from build123d import *

# Parameters (mm, degrees)
F1_DEPTH = 63.5
F4_DEPTH = 16
F5_DEPTH = 13


with BuildPart() as f1:
    # F0 (on Top) → F1 (new body)
    with BuildSketch(Plane.XY):
        with BuildLine():
            Line((-9.75, 5.612486), (-9.75, -5.612486))
            ThreePointArc((-9.75, -5.612486), (0, -11.25), (9.75, -5.612486))
            Line((9.75, -5.612486), (9.75, 5.612486))
            ThreePointArc((9.75, 5.612486), (0, 11.25), (-9.75, 5.612486))
        make_face()
        with BuildLine():
            ThreePointArc((8.75, -5.338539), (0, -10.25), (-8.75, -5.338539))
            Line((-8.75, -5.338539), (-8.75, 5.338539))
            ThreePointArc((-8.75, 5.338539), (0, 10.25), (8.75, 5.338539))
            Line((8.75, 5.338539), (8.75, -5.338539))
        make_face(mode=Mode.SUBTRACT)
    extrude(amount=F1_DEPTH)

    # F3 (on mid) → F4 (join, symmetric)
    with BuildSketch(Plane.XY.offset(31.75)):
        with BuildLine():
            Line((10.45, -5.796551), (10.45, 5.796551))
            ThreePointArc((10.45, 5.796551), (0, 11.95), (-10.45, 5.796551))
            Line((-10.45, 5.796551), (-10.45, -5.796551))
            ThreePointArc((-10.45, -5.796551), (0, -11.95), (10.45, -5.796551))
        make_face()
        with BuildLine():
            ThreePointArc((-9.75, 5.612486), (0, 11.25), (9.75, 5.612486))
            Line((9.75, 5.612486), (9.75, -5.612486))
            ThreePointArc((9.75, -5.612486), (0, -11.25), (-9.75, -5.612486))
            Line((-9.75, -5.612486), (-9.75, 5.612486))
        make_face(mode=Mode.SUBTRACT)
    extrude(amount=F4_DEPTH, both=True)

    # F3 (on mid) → F5 (cut, symmetric)
    with BuildSketch(Plane.XY.offset(31.75)):
        with BuildLine():
            Line((10.45, -5.796551), (10.45, 5.796551))
            ThreePointArc((10.45, 5.796551), (0, 11.95), (-10.45, 5.796551))
            Line((-10.45, 5.796551), (-10.45, -5.796551))
            ThreePointArc((-10.45, -5.796551), (0, -11.95), (10.45, -5.796551))
        make_face()
        with BuildLine():
            ThreePointArc((-9.75, 5.612486), (0, 11.25), (9.75, 5.612486))
            Line((9.75, 5.612486), (9.75, -5.612486))
            ThreePointArc((9.75, -5.612486), (0, -11.25), (-9.75, -5.612486))
            Line((-9.75, -5.612486), (-9.75, 5.612486))
        make_face(mode=Mode.SUBTRACT)
    extrude(amount=F5_DEPTH, both=True, mode=Mode.SUBTRACT)


solid = f1.part
Could you check a few things on this model? Use its own coordinates, in mm. A direction names the side the tool comes from. Give positions to 0.01 mm unless a question says otherwise; leave off trailing zeros. Loops run counter-clockwise (first coordinate to the right, second up) from the corner with the lowest first, then second, coordinate; pieces in that order, holes last. Notation, with made-up numbers: (30, 75.5) -> (86, 75.5) arc R13 cw to (86, 84.5) -> close; hole circle Ø5 at (21, -15). An arc over 180 degrees is marked (long way). Return JSON: item names as keys, results as strings.
Item 1: Which directions (+Z, -Z, +X, -X, +Y, -Y) give clear straight access to the entire face, cutting with the end or side of a thin tool? Please do faces 5 (the flat face through (-9.75, 0, 56)), 6 (the flat face through (-10, -1, 18.75)), 7 (the cylindrical face through (0.15, -10.25, 31.31)), 8 (the flat face through (-10, -1, 47.75)).
Geometry results:
{"face 5": "+Z, -X, +Y, -Y", "face 6": "none", "face 7": "+Z, -Z", "face 8": "+Z"}
Item 2: If we section it at B-B on z = 53: List the corners of the cut face in (x, y) for me, plus the area to 3 significant figures.
Geometry results:
{"outline": "(-9.75, -5.61) arc R11.25 ccw to (9.75, -5.61) -> (9.75, 5.61) arc R11.25 ccw to (-9.75, 5.61) -> close; hole (-8.75, -5.34) arc R10.25 ccw to (8.75, -5.34) -> (8.75, 5.34) arc R10.25 ccw to (-8.75, 5.34) -> close", "area": "66.5 mm²"}
Item 3: We'd pull the mould along Y, two halves only. Please class faces 1 (the flat face through (9.75, 0, 8)), 2 (the cylindrical face through (0.17, 11.25, 55.51)), 3 (the cylindrical face through (-0.17, -11.25, 7.76)), 4 (the flat face through (-8.75, 0, 31)): +Y half, -Y half, draft (parallel to the pull), parting line (faces both ways), or undercut.
Geometry results:
{"face 1": "draft", "face 2": "+Y half", "face 3": "-Y half", "face 4": "undercut"}
Item 4: If we section it at C-C on x = -5: List the corners of the cut face in (y, z) for me.
Geometry results:
{"outline": "(-10.85, 15.75) -> (-10.08, 15.75) -> (-10.08, 0) -> (-8.95, 0) -> (-8.95, 63.5) -> (-10.08, 63.5) -> (-10.08, 47.75) -> (-10.85, 47.75) -> (-10.85, 44.75) -> (-10.08, 44.75) -> (-10.08, 18.75) -> (-10.85, 18.75) -> close; (8.95, 0) -> (10.08, 0) -> (10.08, 15.75) -> (10.85, 15.75) -> (10.85, 18.75) -> (10.08, 18.75) -> (10.08, 44.75) -> (10.85, 44.75) -> (10.85, 47.75) -> (10.08, 47.75) -> (10.08, 63.5) -> (8.95, 63.5) -> close"}
Item 5: If we section it at A-A on y = 2.5: List the corners of the cut face in (x, z) for me.
Geometry results:
{"outline": "(-10.45, 15.75) -> (-9.75, 15.75) -> (-9.75, 0) -> (-8.75, 0) -> (-8.75, 63.5) -> (-9.75, 63.5) -> (-9.75, 47.75) -> (-10.45, 47.75) -> (-10.45, 44.75) -> (-9.75, 44.75) -> (-9.75, 18.75) -> (-10.45, 18.75) -> close; (8.75, 0) -> (9.75, 0) -> (9.75, 15.75) -> (10.45, 15.75) -> (10.45, 18.75) -> (9.75, 18.75) -> (9.75, 44.75) -> (10.45, 44.75) -> (10.45, 47.75) -> (9.75, 47.75) -> (9.75, 63.5) -> (8.75, 63.5) -> close"}
Item 6: I need wall thicknesses on L1, parallel to Y at x = 0, z = 9.5; L2, parallel to X at y = 3.5, z = 38.5; L3, parallel to X at y = 0.5, z = 46. Which ranges of each line are inside material? Lowest first, please. Write a range as from..to.
Geometry results:
{"L1": "y = -11.25..-10.25, 10.25..11.25", "L2": "x = -9.75..-8.75, 8.75..9.75", "L3": "x = -10.45..-8.75, 8.75..10.45"}
Item 7: I'm going to push flat-ended pins straight in: pin 1 (4 mm diameter, centred on y = 8, z = 33, fed in from -X); pin 2 (3 mm diameter, centred on x = 3.5, z = 48, fed in from +Y); pin 3 (3 mm diameter, centred on y = -2, z = 40.5, fed in from +X). Where does each tip first touch, or does it pass through?
Geometry results:
{"pin 1": "stops at x = -9.52", "pin 2": "stops at y = 11.78", "pin 3": "stops at x = 9.75"}
